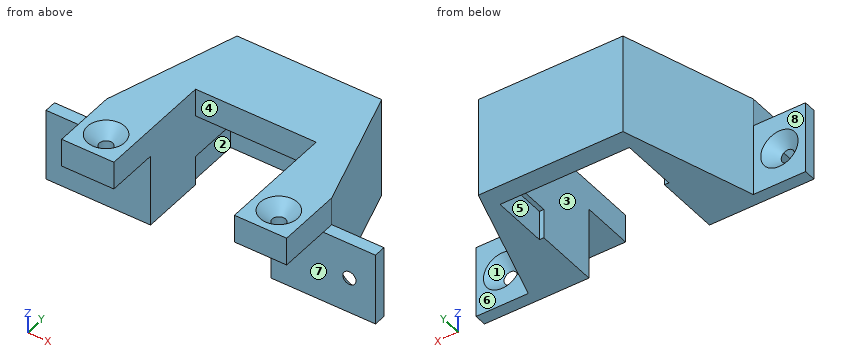
Autodesk Inventor part; units mm, degrees
ref_plane "YZ Plane" through (0, 0, 0) normal (1, 0, 0) x (0, 1, 0)
ref_plane "XZ Plane" through (0, 0, 0) normal (0, 1, 0) x (-1, 0, 0)
ref_plane "XY Plane" through (0, 0, 0) normal (0, 0, 1) x (1, 0, 0)
sketch "Sketch1" plane through (0, 0, 0) normal (0, 1, 0) x (-1, 0, 0)
  line L0 (0, 0) -> (-30, 0)
  line L1 (-30, 0) -> (-30, -10.6)
  line L2 (-30, -10.6) -> (0, -10.6)
  line L3 (0, -10.6) -> (0, 0)
  line L4 (0, -10.6) -> (1.1, -10.6)
  line L5 (1.1, -10.6) -> (1.1, -18)
  line L6 (1.1, -18) -> (0, -18)
  line L7 (0, -18) -> (0, -10.6)
  line L8 (-30, -10.6) -> (-31.1, -10.6)
  line L9 (-31.1, -10.6) -> (-31.1, -18)
  line L10 (-31.1, -18) -> (-30, -18)
  line L11 (-30, -18) -> (-30, -10.6)
  line L12 (0, -18) -> (-30, -18)
  dimension "d0" = 30
  dimension "d1" = 10.6
  dimension "d2" = 1.1
  dimension "d3" = 1.1
  dimension "d4" = 7.4
  dimension "d5" = 7.4
extrude "Extrusion1" add sketch "Sketch1" along normal blind 3
sketch "Sketch2" plane through (30, 0, 0) normal (1, 0, 0) x (0, 0, -1)
  point P0 (0, 0)
sketch "Sketch3" plane through (30, 0, 0) normal (1, 0, 0) x (0, 0, -1)
  line L0 (0, 0) -> (10.6, 0)
  line L1 (0, 0) -> (0, -30)
  line L2 (0, -30) -> (10.6, -30)
  line L3 (10.6, 0) -> (10.6, -30)
  line L4 (10.6, 0) -> (0, 0)
  line L5 (0, 0) -> (10.6, 0)
  dimension "d8" = 30
sketch "Sketch4" plane through (31.1, 0, -10.6) normal (1, 0, 0) x (0, 0, -1)
  line L0 (0, 0) -> (7.4, 0)
  line L1 (7.4, 0) -> (7.4, -14)
  line L2 (7.4, -14) -> (0, -14)
  line L3 (0, -14) -> (0, 0)
  line L4 (0, 0) -> (7.4, 0)
  point P0 (-10.6, 0)
  dimension "d9" = 14
extrude "Extrusion2" add sketch "Sketch3" along normal blind 3
extrude "Extrusion3" add sketch "Sketch4" along normal blind 3
sketch "Sketch5" plane through (31.1, -14, -18) normal (0, -1, 0) x (1, 0, 0)
  line L0 (1.9, 7.4) -> (1.9, 18)
  line L1 (1.9, 7.4) -> (1.9, 0)
  line L2 (0, 0) -> (3, 0)
  line L3 (-1.1, 18) -> (-1.1, 7.4)
  line L4 (-1.1, 7.4) -> (-1.1, 0)
  line L5 (0, 0) -> (-32.2, 0)
  line L6 (-1.1, 7.4) -> (1.9, 7.4)
  line L7 (1.9, 7.4) -> (-1.1, 7.4)
  point P0 (-31.1, 18)
extrude "Extrusion4" add sketch "Sketch5" along normal blind 16
sketch "Sketch6" plane through (30, 0, 0) normal (0, 1, 0) x (1, 0, 0)
  line L0 (1.1, 10.6) -> (1.1, 18)
  line L1 (1.1, 10.6) -> (1.1, 0)
  line L2 (0, 0) -> (3, 0)
  line L3 (1.1, 0) -> (0, 0)
  line L4 (0, 0) -> (0, 10.6)
  line L5 (0, 0) -> (0, 18)
  line L6 (0, 10.6) -> (1.1, 10.6)
  line L7 (1.1, 10.6) -> (0, 10.6)
  point P0 (-30, 0)
extrude "Extrusion5" add sketch "Sketch6" along normal blind 3
sketch "Sketch7" plane through (31.1, 3, 0) normal (1, 0, 0) x (0, 0, -1)
  point P0 (0, -3)
sketch "Sketch8" plane through (31.1, 0, 0) normal (0, 1, 0) x (1, 0, 0)
  line L0 (0, 0) -> (1.9, 0)
  line L1 (0, 0) -> (0, 18)
  line L2 (1.9, 0) -> (0, 0)
  line L3 (0, 0) -> (0, 18)
  line L4 (0, 18) -> (1.9, 18)
  line L5 (1.9, 18) -> (1.9, 0)
  point P0 (-31.1, 0)
extrude "Extrusion6" add sketch "Sketch8" along normal up to surface (3 mm away)
sketch "Sketch9" plane through (33, -14, -10.6) normal (0, 0, 1) x (1, 0, 0)
  line L0 (0, 0) -> (0, 14)
  line L1 (0, 0) -> (1.1, 0)
  line L2 (1.1, 14) -> (1.1, 0)
  line L3 (0, 14) -> (1.1, 14)
  line L4 (0, 0) -> (0, 14)
  line L5 (0, 14) -> (1.1, 14)
  line L6 (1.1, 14) -> (1.1, 0)
  line L7 (1.1, 0) -> (0, 0)
  line L8 (0, 0) -> (0, 14)
  point P0 (-33, 14)
extrude "Extrusion7" cut sketch "Sketch9" against normal blind 2000
sketch "Sketch10" plane through (33, 0, 0) normal (1, 0, 0) x (0, 0, -1)
  line L0 (0, -30) -> (0, 3)
  line L1 (0, -30) -> (18, -30)
  line L2 (18, -30) -> (18, -27)
  line L3 (18, -27) -> (0, -27)
  line L4 (0, -27) -> (0, -30)
  point P0 (0, 0)
  point P1 (0, 1.1)
  dimension "d25" = 18
  dimension "d26" = 3
extrude "Extrusion8" add sketch "Sketch10" along normal blind 14
sketch "Sketch12" plane through (0, 3, 0) normal (0, 1, 0) x (1, 0, 0)
  line L0 (0, 10.6) -> (0, 0)
  line L1 (15, 0) -> (15, 18)
  point P0 (30, 10.6)
  point P1 (31.1, 10.6)
  point P2 (30, 0)
ref_plane "Work Plane1" through (15, 0, -10.6) normal (-1, 0, 0) x (0, 0, 1)
mirror "Mirror1" about plane through (15, 0, -10.6) normal (-1, 0, 0) of "Extrusion2", "Extrusion3", "Extrusion4", "Extrusion5", "Extrusion6", "Extrusion7", "Extrusion8"
sketch "Sketch13" plane through (30, -30, 0) normal (0, 0, 1) x (1, 0, 0)
  line L0 (-33, 33) -> (3, 33)
  line L1 (-30, 30) -> (0, 30)
  line L2 (0, 30) -> (0, 33)
  line L3 (0, 33) -> (-30, 33)
  line L4 (-30, 33) -> (-30, 30)
  point P0 (-31.1, 33)
  point P1 (1.1, 33)
  dimension "d36" = 30
extrude "Extrusion10" add sketch "Sketch13" along normal blind 7
sketch "Sketch14" plane through (0, 0, 0) normal (0, -1, 0) x (1, 0, 0)
  line L0 (0, 0) -> (0, 7)
  line L1 (30, 0) -> (30, -10.6)
  line L2 (0, 7) -> (30, 7)
  line L3 (30, 7) -> (30, 0)
  line L4 (30, 0) -> (0, 0)
  line L5 (0, 0) -> (0, 7)
extrude "Extrusion11" add sketch "Sketch14" along normal blind 14
sketch "Sketch16" plane through (0, 3, 0) normal (0, 1, 0) x (1, 0, 0)
  line L0 (30, -7) -> (0, -7)
  line L1 (-3, 18) -> (33, 18)
  line L2 (30, -7) -> (0, -7)
  line L3 (0, -7) -> (0, 18)
  line L4 (0, 18) -> (30, 18)
  line L5 (30, 18) -> (30, -7)
  line L6 (33, 18) -> (31.1, 18)
  line L7 (31.1, 18) -> (30, 18)
  line L8 (30, 18) -> (30, 0)
  line L9 (30, 0) -> (31.1, 0)
  line L10 (0, 0) -> (0, 18)
  line L11 (0, 18) -> (-1.1, 18)
  line L12 (-1.1, 0) -> (0, 0)
  line L13 (0, 0) -> (0, 18)
  line L14 (31.1, 18) -> (33, 18)
  line L15 (33, 0) -> (31.1, 0)
  line L16 (33, 0) -> (30, 0)
  line L17 (31.1, 18) -> (-1.1, 18)
  line L18 (-3, 18) -> (-17, 18)
  line L19 (-1.1, 18) -> (-3, 18)
  line L20 (-3, 18) -> (-3, 0)
  line L21 (-3, 18) -> (-3, 0)
  line L22 (-3, 0) -> (-1.1, 0)
  line L23 (0, 0) -> (-3, 0)
  line L24 (33, 18) -> (33, 0)
  line L25 (33, 18) -> (33, 0)
extrude "Extrusion13" add sketch "Sketch16" along normal blind 2
sketch "Sketch17" plane through (30, -30, 0) normal (0, 0, 1) x (1, 0, 0)
  line L0 (0, 35) -> (3, 35)
  line L1 (3, 35) -> (0, 35)
  line L2 (0, 35) -> (0, 0)
  line L3 (0, 0) -> (3, 0)
  line L4 (3, 0) -> (3, 35)
  line L5 (0, 0) -> (17, 0)
  line L6 (0, 0) -> (13, 0)
  line L7 (13, 0) -> (13, -13.0001)
  line L8 (13, -13.0001) -> (0, -13.0001)
  line L9 (0, -13.0001) -> (0, 0)
  point P0 (-30, 30)
  dimension "d45" = 13
extrude "Extrusion14" add sketch "Sketch17" along normal blind 7 contours L0 L4 L3 L2
sketch "Sketch18" plane through (33, -30, 0) normal (0, 0, 1) x (1, 0, 0)
  line L0 (-3, 16) -> (-3, 0)
  line L1 (-3, 0) -> (10, 0)
  line L2 (10, 0) -> (10, -13)
  line L3 (10, -13) -> (-3, -13)
  line L4 (-3, -13) -> (-3, 0)
  point P0 (-33, 30)
  dimension "d48" = 13
  dimension "d49" = 13
extrude "Extrusion15" add sketch "Sketch18" along normal blind 7
sketch "Sketch19" plane through (33, -30, 0) normal (0, 1, 0) x (1, 0, 0)
  line L0 (10, 0) -> (10, -7)
  line L1 (10, -7) -> (0, -7)
  line L2 (10, 0) -> (0, 0)
  line L3 (0, 0) -> (0, -7)
  line L4 (0, -7) -> (10, -7)
  line L5 (10, -7) -> (10, 0)
  point P0 (-33, 0)
sketch "Sketch20" plane through (30, -30, 7) normal (0, 0, 1) x (1, 0, 0)
  line L0 (13, -13) -> (13, 0)
  line L1 (13, -6.5) -> (0, -6.5) construction
  line L2 (0, -13) -> (0, 0)
  line L3 (3, 0) -> (13, 0)
  line L4 (6.5, 0) -> (6.5, -6.5) construction
  circle A0 centre (6.5, -6.5) radius 1.65
  point P0 (-30, 30)
  dimension "d52" = 3.3
extrude "Extrusion16" cut sketch "Sketch20" against normal blind 7
chamfer "Chamfer3" distance 3 angle 45 1 edges at (34.85, -36.5, 7)
extrude "Extrusion17" add sketch "Sketch19" along normal blind 3
sketch "Sketch21" plane through (33, -27, -18) normal (0, 1, 0) x (1, 0, 0)
  line L0 (14, 0) -> (14, -18)
  line L1 (14, 0) -> (23, 0)
  line L2 (23, 0) -> (23, -18)
  line L3 (23, -18) -> (14, -18)
  line L4 (14, -18) -> (14, 0)
  point P0 (-33, -18)
  dimension "d60" = 9
extrude "Extrusion18" add sketch "Sketch21" against normal blind 3
sketch "Sketch22" plane through (33, -27, 7) normal (0, 1, 0) x (1, 0, 0)
  line L0 (10, 7) -> (23, 7)
  line L1 (16.5, 7) -> (16.5, 25) construction
  line L2 (0, 25) -> (23, 25)
  line L3 (23, 25) -> (23, 7)
  line L4 (23, 16) -> (16.5, 16) construction
  circle A0 centre (16.5, 16) radius 1.65
  point P0 (-33, 7)
  dimension "d63" = 3.3
extrude "Extrusion19" cut sketch "Sketch22" against normal blind 3
chamfer "Chamfer4" distance 3 angle 45 1 edges at (47.85, -27, -9)
sketch "Sketch24" plane through (30, -30, 7) normal (0, 0, 1) x (1, 0, 0)
  line L0 (1.1, 30) -> (1.1, 16)
  line L1 (-30, 35) -> (3, 35)
  line L2 (-30, 16) -> (-30, 35)
  line L3 (0, 16) -> (-30, 16)
  line L4 (0, 16) -> (0, -13)
  line L5 (0, -13) -> (13, -13)
  line L6 (13, -13) -> (13, 3)
  line L7 (3, 3) -> (13, 3)
  line L8 (3, 3) -> (3, 35)
  circle A0 centre (6.5, -6.5) radius 4.65
  line L9 (3, 35) -> (3, 3)
  line L10 (3, 35) -> (3, 3)
  line L11 (3, 3) -> (13, 3)
  line L12 (3, 35) -> (13, 3)
  point P0 (-30, 30)
extrude "Extrusion20" add sketch "Sketch24" against normal blind 25 contours L12 L7 L8
ref_plane "Work Plane2" through (15, 0, 0) normal (1, 0, 0) x (0, 0, -1)
mirror "Mirror2" about plane through (15, 0, 0) normal (1, 0, 0) of "Extrusion1", "Extrusion2", "Extrusion3", "Extrusion4", "Extrusion5", "Extrusion6", "Extrusion7", "Extrusion8", "Extrusion10", "Extrusion11", "Extrusion13", "Extrusion14", "Extrusion15", "Extrusion16", "Chamfer3", "Extrusion17", "Extrusion18", "Extrusion19", "Chamfer4", "Extrusion20"
ref_plane "Work Plane3" through (15, 0, -10.6) normal (-1, 0, 0) x (0, 0, 1)
properties part number "buttonHolder"
For this review, take the finished solid that the model builds, in its own axes (mm). Face numbers are marked on the shaded views. A direction names the side the tool comes from. Coordinates: 2 decimals unless noted, no trailing zeros. Loops run counter-clockwise (first coordinate to the right, second up) from the corner with the lowest first, then second, coordinate; pieces in that order, holes last. Notation, with made-up numbers: (-23.5, 23) -> (6.5, 23) arc R6 ccw to (6.5, 32) -> close; hole circle Ø7 at (36.5, 74). An arc over 180 degrees is marked (long way). Write each question's results on one line, items separated by ' | '.
Q1. Add section C-C, the plane z = 1.75. State the section outline as (x, y) points, then the cut area to 3 significant figures.
Taken from the geometry:
outline: (-13, -43) -> (0, -43) -> (0, -14) -> (30, -14) -> (30, -43) -> (43, -43) -> (43, -27) -> (33, 5) -> (-3, 5) -> (-13, -27) -> close; hole circle Ø3.3 at (-6.5, -36.5); hole circle Ø3.3 at (36.5, -36.5) | area: 1,480 mm²
Q2. Mouldability with a two-part tool opening along Y and no side actions: class the marked faces 1, 2 and 3 as +Y half, -Y half, draft (parallel to the pull), parting line (faces both ways), or undercut.
Taken from the geometry:
face 1: +Y half | face 2: undercut | face 3: draft
Q3. Add section D-D, the plane y = -36.5. State the section outline as (x, z) points.
Taken from the geometry:
outline: (-13, 0) -> (-8.15, 0) -> (-8.15, 4) -> (-11.15, 7) -> (-13, 7) -> close; (-4.85, 0) -> (0, 0) -> (0, 7) -> (-1.85, 7) -> (-4.85, 4) -> close; (30, 0) -> (34.85, 0) -> (34.85, 4) -> (31.85, 7) -> (30, 7) -> close; (38.15, 0) -> (43, 0) -> (43, 7) -> (41.15, 7) -> (38.15, 4) -> close
Q4. For pin 1 Ø0.9 at (x, y) = (-21.5, -28) entering from +Z; pin 2 Ø10 at (x, y) = (7.5, -14.5) entering from -Z; pin 3 Ø10 at (y, z) = (-37.5, 1) entering from -X; pin 4 Ø12 at (y, z) = (-23, -6.5) entering from -X, all flat-tipped, find the tip position at first contact; note any pin that passes through.
Taken from the geometry:
pin 1: z = 0 | pin 2: z = 0 | pin 3: x = -13 | pin 4: x = -26
Q5. Add section B-B, the plane y = -19. State the section outline as (x, z) points.
Taken from the geometry:
outline: (-10.5, -18) -> (0, -18) -> (0, 7) -> (-10.5, 7) -> close; (30, -18) -> (40.5, -18) -> (40.5, 7) -> (30, 7) -> close
Q6. Machinability: for the marked faces 4, 5, 6, 7 and 8, which of the approach directions +Z, -Z, +X, -X, +Y, -Y give a long, thin tool a straight path to every point of the face, cutting with its end or side? Answer none if there is none.
Taken from the geometry:
face 4: +Z, -Z, -Y | face 5: -Z | face 6: +Z, -Z, +X, +Y | face 7: -Z, +X, -X, -Y | face 8: +Z, -Z, -X, +Y
Q7. To check wall thickness, follow line 1 along X through (y, z) = (-28.5, 0.25); line 2 along X through (y, z) = (-29.95, -9); line 3 along X through (y, z) = (-29, -8). State the ranges of each line that lie inside material, in increasing order. Write a range as [from, to].
Taken from the geometry:
line 1: [-13, 0], [30, 43] | line 2: [-26, -21.2], [-17.8, 0], [30, 47.8], [51.2, 56] | line 3: [-26, -21.95], [-17.05, 0], [30, 47.05], [51.95, 56]
